For this review, take the finished solid that the model builds, in its own axes (mm). A direction names the side the tool comes from. Give positions to 0.01 mm unless a question says otherwise; leave off trailing zeros. Write each loop counter-clockwise with the first axis right and the second up, starting at its lowest first coordinate (ties: lowest second). Pieces come first, ordered by that corner, then holes.
from build123d import *

# Parameters (mm, degrees)
REVOLVE1_ANGLE      = 180
SKETCH4_R           = 25
BOSS_EXTRUDE1_DEPTH = 10
SKETCH5_R           = 35
BOSS_EXTRUDE2_DEPTH = 10


# Read off the part's stored shape, not the designer's step: Revolve1
with BuildPart() as part:
    # Revolve1 outline → Revolve1 (revolve)
    with BuildSketch(Plane(origin=(0, 0, 0), x_dir=(0, -1, 0), z_dir=(0, 0, 1))):
        with BuildLine():
            Line((0, -75), (0, -85))
            ThreePointArc((0, -85), (24.748737342, -74.748737342), (35, -50))
            Line((35, -50), (35, 0))
            Line((35, 0), (0, 0))
            Line((0, 0), (0, -25))
            ThreePointArc((0, -25), (25, -50), (0, -75))
        make_face()
    revolve(axis=Axis((0, 0, 0), (1, 0, 0)), revolution_arc=REVOLVE1_ANGLE)

    # Sketch4 → Boss-Extrude1 (add)
    with BuildSketch(Plane(origin=(0, 0, 0), x_dir=(0, 0, -1), z_dir=(1, 0, 0))):
        with Locations(Location((0, 0, 0), (0, 0, 270))):
            Circle(SKETCH4_R)
    extrude(amount=BOSS_EXTRUDE1_DEPTH)

    # Sketch5 → Boss-Extrude2 (add)
    with BuildSketch(Plane(origin=(0, 0, 0), x_dir=(0, 0, -1), z_dir=(1, 0, 0))):
        with Locations(Location((0, 0, 0), (0, 0, 180))):
            Circle(SKETCH5_R)
    extrude(amount=-BOSS_EXTRUDE2_DEPTH)


solid = part.part
(1) For L1, parallel to X at y = 14, z = 31; L2, parallel to X at y = 6, z = 7; L3, parallel to X at y = -9, z = -11.5, list the stretches that pass through material, from the lowest coordinate up.
(2) We need section C-C (x = -1.5). Write out the cut boundary in (y, z).
(3) Tool access review of faces 1 (the flat face through (0, -24, -8)), 2 (the cylindrical face through (-19.094, -1.539, -34.966)), 3 (the flat face through (-10, 0, 13)): name each direction out of +Z, -Z, +X, -X, +Y, -Y from which nothing blocks a thin tool from reaching the whole face with its end or side.
(4) We need section B-B (y = 0). Write out the cut boundary in (x, z), and give its area (3 significant figures).
(5) Clearance check with flat-ended pins moving along their axes: pin 1 Ø10 at (x, y) = (-51, -9.5) entering from +Z; pin 2 Ø10 at (x, y) = (-13, 7) entering from -Z; pin 3 Ø4 at (x, y) = (-72, 1.5) entering from -Z. State where each tip first meets the part, or that it passes through.
(6) We need section A-A (z = -21). Write out the cut boundary in (x, y), and give its area (3 significant figures).
(7) We need section D-D (y = 15.5). Write out the cut boundary in (x, z), and give its area (3 significant figures).
The answers:
1. L1: x = -10 to 0
1. L2: x = -10 to 10
1. L3: x = -81.81 to -70.29, -29.71 to 10
2. outline: circle Ø70 at (0, 0)
3. face 1: +X
3. face 2: +X, -X
3. face 3: +Z, -X, +Y, -Y
4. outline: (-85, 0) arc R35 ccw to (-50, -35) - (0, -35) - (0, -25) - (10, -25) - (10, 25) - (0, 25) - (0, 35) - (-10, 35) - (-10, 0) - (-25, 0) arc R25 cw to (-75, 0) - close
4. area: 2,580 mm2
5. pin 1: stops at z = -20.33
5. pin 2: stops at z = -34.94
5. pin 3: stops at z = -28.69
6. outline: (-50, -28) - (0, -28) - (0, -13.56) - (10, -13.56) - (10, 13.56) - (0, 13.56) - (0, 28) - (-50, 28) arc R28 ccw to start; hole circle Ø27.13 at (-50, 0)
6. area: 3,720 mm2
7. outline: (-81.38, 0) arc R31.38 ccw to (-50, -31.38) - (0, -31.38) - (0, -19.62) - (10, -19.62) - (10, 19.62) - (0, 19.62) - (0, 31.38) - (-10, 31.38) - (-10, 0) - (-30.38, 0) arc R19.62 cw to (-69.62, 0) - close
7. area: 2,440 mm2
